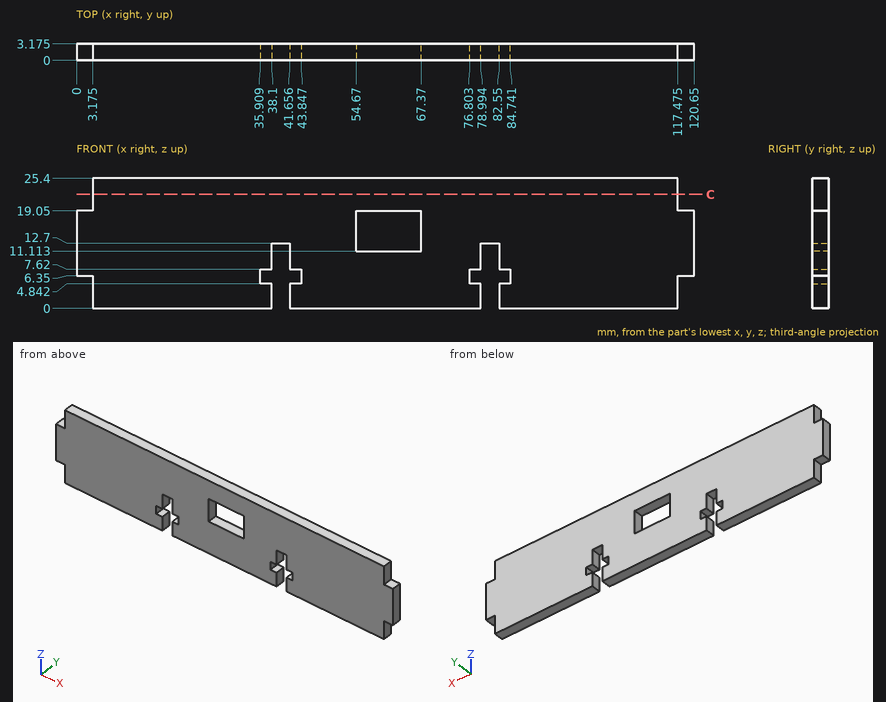
Print and shaded views of the part. All mm, measured from the part's lowest x, y and z. Round coordinates to 2 decimals unless told otherwise and drop trailing zeros. Write each loop counter-clockwise with the first axis right and the second up, starting at its lowest first coordinate (ties: lowest second). Pieces come first, ordered by that corner, then holes.
(1) Slice it at C-C, the plane z = 22.25. Write the cut outline in (x, y) (1 decimal).
(2) Probe line 1 along X through (y, z) = (1.7, 5.75) (1 decimal); line 2 along X through (y, z) = (2.7, 17); line 3 along Z through (x, y) = (36.5, 1.75). List the from-to ranges inside material, lowest first.
(3) Drop flat-ended pins along their axis: P1, Ø1, axis at y = 1, z = 13.5, coming from the -X side; P2, Ø1, axis at y = 1.5, z = 1.5, coming from the -X side (1 decimal); P3, Ø1.6, axis at y = 2.5, z = 22.5, coming from the +X side (1 decimal). Give the stop position or say it passes through.
From the geometry:
1. outline: (3.2, 0) - (117.5, 0) - (117.5, 3.2) - (3.2, 3.2) - close
2. line 1: x = 3.2 to 35.9, 43.8 to 76.8, 84.7 to 117.5
2. line 2: x = 0 to 54.67, 67.37 to 120.65
2. line 3: z = 0 to 4.84, 7.62 to 25.4
3. P1: stops at x = 0
3. P2: stops at x = 3.2
3. P3: stops at x = 117.5
